Autodesk Inventor part; units mm, degrees
ref_plane "YZ Plane" through (0, 0, 0) normal (1, 0, 0) x (0, 1, 0)
ref_plane "XZ Plane" through (0, 0, 0) normal (0, 1, 0) x (-1, 0, 0)
ref_plane "XY Plane" through (0, 0, 0) normal (0, 0, 1) x (1, 0, 0)
sketch "Sketch1" plane through (0, 0, 0) normal (0, 0, 1) x (1, 0, 0)
  line L0 (0, 14.6647) -> (12.7, 7.3323)
  line L1 (12.7, 7.3323) -> (12.7, -7.3323)
  line L2 (12.7, -7.3323) -> (0, -14.6647)
  line L3 (0, -14.6647) -> (-12.7, -7.3323)
  line L4 (-12.7, -7.3323) -> (-12.7, 7.3323)
  line L5 (-12.7, 7.3323) -> (0, 14.6647)
  point P0 (0, 0)
  point P1 (0, 0)
  dimension "d0" = 25.4
extrude "Extrusion1" add sketch "Sketch1" along normal blind 6.35
sketch "Sketch2" plane through (0, 0, 6.35) normal (0, 0, 1) x (1, 0, 0)
  line L0 (12.7, 7.3323) -> (0, 14.6647)
  line L1 (0, 14.6647) -> (-12.7, 7.3323)
  line L2 (-12.7, 7.3323) -> (-12.7, -7.3323)
  line L3 (-12.7, -7.3323) -> (0, -14.6647)
  line L4 (0, -14.6647) -> (12.7, -7.3323)
  line L5 (12.7, -7.3323) -> (12.7, 7.3323)
  line L6 (7.5523, 0) -> (3.7762, -6.5405)
  line L7 (3.7762, -6.5405) -> (-3.7762, -6.5405)
  line L8 (-3.7762, -6.5405) -> (-7.5523, 0)
  line L9 (-7.5523, 0) -> (-3.7762, 6.5405)
  line L10 (-3.7762, 6.5405) -> (3.7762, 6.5405)
  line L11 (3.7762, 6.5405) -> (7.5523, 0)
  line L12 (3.7762, 6.5405) -> (12.7, 6.5405)
  line L13 (3.7762, -6.5405) -> (12.7, -6.5405)
  point P0 (0, 0)
  point P1 (0, 0)
  dimension "d3" = 13.081
extrude "Extrusion2" add sketch "Sketch2" along normal blind 9.525 contours L5 L12 L10 L9 L8 L7 L13 L4 L3 L2 L1 L0
sketch "Sketch3" plane through (0, 0, 15.875) normal (0, 0, 1) x (1, 0, 0)
  line L0 (12.7, 7.3323) -> (0, 14.6647)
  line L1 (0, 14.6647) -> (-12.7, 7.3323)
  line L2 (-12.7, 7.3323) -> (-12.7, -7.3323)
  line L3 (-12.7, -7.3323) -> (0, -14.6647)
  line L4 (0, -14.6647) -> (12.7, -7.3323)
  line L5 (12.7, -7.3323) -> (12.7, -6.5405)
  line L6 (12.7, -6.5405) -> (-3.7762, -6.5405)
  line L7 (-3.7762, -6.5405) -> (-7.5523, 0)
  line L8 (-7.5523, 0) -> (-3.7762, 6.5405)
  line L9 (-3.7762, 6.5405) -> (12.7, 6.5405)
  line L10 (12.7, 6.5405) -> (12.7, 7.3323)
  line L11 (12.7, 6.5405) -> (12.7, -6.5405)
  point P0 (0, 0)
extrude "Extrusion3" add sketch "Sketch3" along normal blind 6.35
sketch "Sketch4" plane through (0, 0, 0) normal (0, 0, -1) x (-1, 0, 0)
  circle A0 centre (0, 0) radius 12.7
  line L0 (0, 14.6647) -> (-12.7, 7.3323)
extrude "Extrusion4" cut sketch "Sketch4" against normal through all draft 30 keep common part
sketch "Sketch5" plane through (0, 0, 0) normal (0, 0, -1) x (-1, 0, 0)
  circle A0 centre (0, 0) radius 12.7
  circle A1 centre (0, 0) radius 4.3656
  arc A2 (-12.7, 0) -> (-6.35, -10.9985) centre (0, 0) ccw
  arc A3 (-6.35, -10.9985) -> (6.35, -10.9985) centre (0, 0) ccw
  arc A4 (6.35, -10.9985) -> (12.7, 0) centre (0, 0) ccw
  arc A5 (12.7, 0) -> (6.35, 10.9985) centre (0, 0) ccw
  arc A6 (6.35, 10.9985) -> (-6.35, 10.9985) centre (0, 0) ccw
  arc A7 (-6.35, 10.9985) -> (-12.7, 0) centre (0, 0) ccw
  dimension "d13" = 8.7312
extrude "Extrusion5" cut sketch "Sketch5" against normal up to next contours A1
fillet "Fillet1" radius 3.175 6 edges at (12.7, 0, 22.225) (6.35, 10.9985, 22.225) (-6.35, 10.9985, 22.225) (-12.7, 0, 22.225) (-6.35, -10.9985, 22.225) (6.35, -10.9985, 22.225)
properties part number "bottom nut"
Work out the finished part from the listing and answer in its coordinate system (mm). A direction names the side the tool comes from. Coordinates: 2 decimals unless noted, no trailing zeros. Write each loop counter-clockwise with the first axis right and the second up, starting at its lowest first coordinate (ties: lowest second). Pieces come first, ordered by that corner, then holes. Notation, with made-up numbers: M 1.5,61.25 L 45.5,61.25 A33 cw 45.5,89.25 Z; hole C 12.25,33.5 d3. An arc over 180 degrees is marked long. Use one line per item in the form item = value. Start each with the question number.
1. Straight lines are drawn through the part: probe 1 along Z at (x, y) = (-1.25, 5) (3 decimals); probe 2 along Y at (x, z) = (0, 4.5); probe 3 along Y at (x, z) = (6.5, 10). For each, find the intervals that lie inside material, in ascending order. Write a range as from..to.
2. Each of these flat-tipped pins is pushed along its axis until it touches: P1, Ø5, axis at x = 0, y = 0, coming from the -Z side (3 decimals); P2, Ø3, axis at x = 9.5, y = -10.5, coming from the +Z side; P3, Ø8, axis at x = 2, z = 14, coming from the -Y side. Where does it stop, or does it pass through?
3. A tool of negligible diameter and unlimited length cuts with its end or side. For faces 1 (the face through (11.43, 6.56, 0.83)), 2 (the face through (5, 0, 6.35)), from which of +Z, -Z, +X, -X, +Y, -Y can it reach the whole face along a straight path? Write none if from no direction.
4. The part is cut by section A-A (z = 10). Give the vertices of the cut face in (x, y), plus the area to 3 significant figures.
5. The mould has two halves that part along Z. Classify faces 3 (the face through (0.03, 13.18, 0.83)), 4 (the face through (5.784, 10.223, 21.32)), 5 (the face through (-5.691, 3.224, 11.046)): released by +Z, released by -Z, zero draft, split by the parting line, or undercut.
Evaluation:
q1.probe_1 = 0..6.35, 15.875..22.225
q1.probe_2 = -14.66..-4.37, 4.37..14.66
q1.probe_3 = -10.91..-6.54, 6.54..10.91
q2.P1 = 15.875
q2.P2 = 20.51
q2.P3 = -14.66
q3.face_1 = -Z, +X, +Y
q3.face_2 = +X
q4.outline = M -12.7,-7.33 L 0,-14.66 L 12.7,-7.33 L 12.7,-6.54 L -3.78,-6.54 L -7.55,0 L -3.78,6.54 L 12.7,6.54 L 12.7,7.33 L 0,14.66 L -12.7,7.33 Z
q4.area = 319 mm^2
q5.face_3 = released by -Z
q5.face_4 = released by +Z
q5.face_5 = undercut
